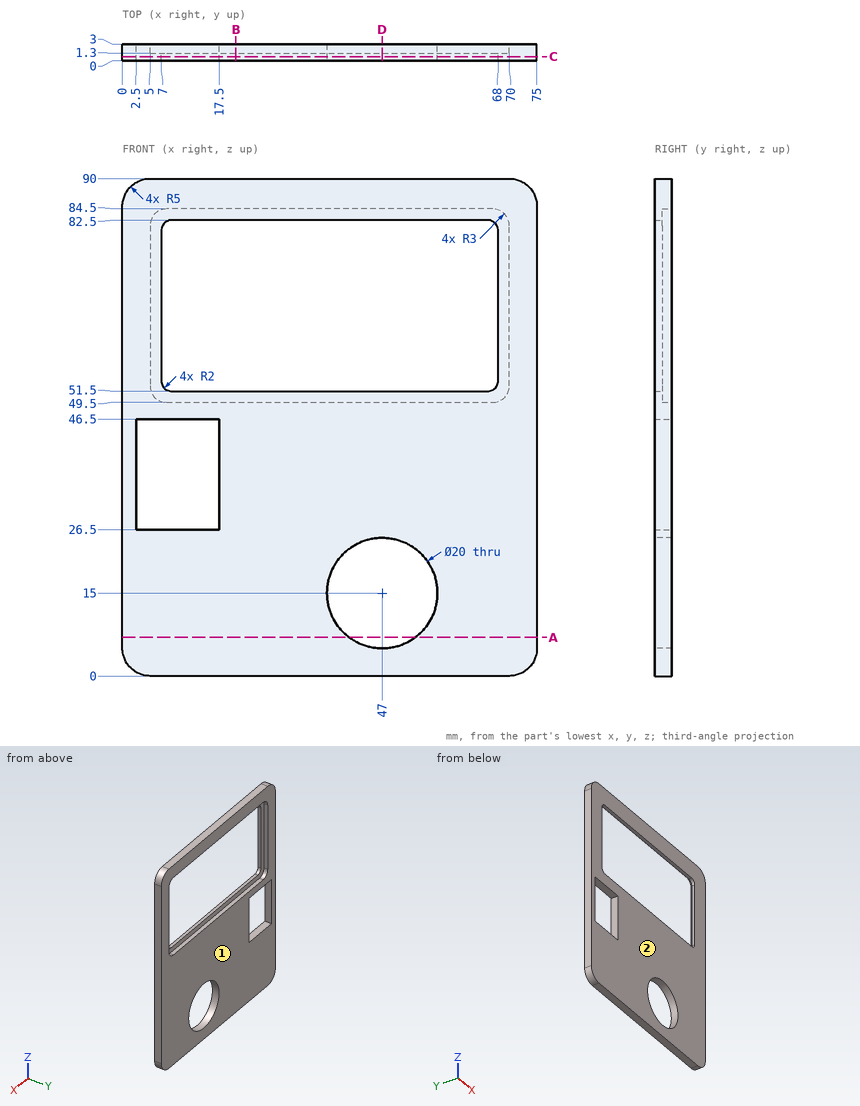
Study the drawing (mm; zero at the part's minimum x, y, z) and answer. Give positions to 0.01 mm unless a question says otherwise; leave off trailing zeros. Write each loop counter-clockwise with the first axis right and the second up, starting at its lowest first coordinate (ties: lowest second). Pieces come first, ordered by that corner, then holes. Notation, with made-up numbers: (3.25, -11.5) -> (34.25, -11.5) arc R6 cw to (34.25, -3.5) -> close; hole circle Ø9 at (68, -24.5). An arc over 180 degrees is marked (long way). Write item = value, one per line.
Q1. Section A-A on z = 7 is taken. Determine the outline of the cut face in (x, y), and give its area (3 significant figures).
Computed values:
outline = (0, 0) -> (41, 0) -> (41, 3) -> (0, 3) -> close; (53, 0) -> (75, 0) -> (75, 3) -> (53, 3) -> close
area = 189 mm^2
Q2. Section C-C on y = 0.7 is taken. Determine the outline of the cut face in (x, z), and give its area (3 significant figures).
Computed values:
outline = (0, 5) arc R5 ccw to (5, 0) -> (70, 0) arc R5 ccw to (75, 5) -> (75, 85) arc R5 ccw to (70, 90) -> (5, 90) arc R5 ccw to (0, 85) -> close; hole (2.5, 26.5) -> (17.5, 26.5) -> (17.5, 46.5) -> (2.5, 46.5) -> close; hole (7, 53.5) arc R2 ccw to (9, 51.5) -> (66, 51.5) arc R2 ccw to (68, 53.5) -> (68, 80.5) arc R2 ccw to (66, 82.5) -> (9, 82.5) arc R2 ccw to (7, 80.5) -> close; hole circle Ø20 at (47, 15)
area = 4,230 mm^2
Q3. Flat-ended cylindrical pins translate along their axes: pin 1 Ø17.5 at (x, z) = (47.5, 75.5) entering from +Y; pin 2 Ø16 at (x, z) = (47, 15) entering from +Y. Find the tip coordinate at first contact, or state that the pin passes through.
Computed values:
pin_1 = 1.3
pin_2 = through
Q4. Consider line 1 along Z through (x, y) = (47, 1.2); line 2 along Z through (x, y) = (15, 2.3); line 3 along X through (y, z) = (1.1, 15). Determine where each line is inside the solid, lowest interval first.
Computed values:
line_1 = 0 to 5, 25 to 51.5, 82.5 to 90
line_2 = 0 to 26.5, 46.5 to 49.5, 84.5 to 90
line_3 = 0 to 37, 57 to 75
Q5. Section D-D on x = 47 is taken. Determine the outline of the cut face in (y, z), and give its area (3 significant figures).
Computed values:
outline = (0, 0) -> (3, 0) -> (3, 5) -> (0, 5) -> close; (0, 25) -> (3, 25) -> (3, 49.5) -> (1.3, 49.5) -> (1.3, 51.5) -> (0, 51.5) -> close; (0, 82.5) -> (1.3, 82.5) -> (1.3, 84.5) -> (3, 84.5) -> (3, 90) -> (0, 90) -> close
area = 110 mm^2
Q6. Section B-B on x = 20.5 is taken. Determine the outline of the cut face in (y, z).
Computed values:
outline = (0, 0) -> (3, 0) -> (3, 49.5) -> (1.3, 49.5) -> (1.3, 51.5) -> (0, 51.5) -> close; (0, 82.5) -> (1.3, 82.5) -> (1.3, 84.5) -> (3, 84.5) -> (3, 90) -> (0, 90) -> close
Q7. For a pull along Y with two mould halves and no side action, classify the marked faces 1 and 2 as pulls with the +Y half, pulls with the -Y half, needs draft (parallel to the pull), parting line crosses it, or undercut.
Computed values:
face_1 = pulls with the +Y half
face_2 = pulls with the -Y half
